Verification items for this drawing (mm, ordinates from the low corner). A direction names the side the tool comes from. Coordinates: 2 decimals unless noted, no trailing zeros. Loops run counter-clockwise (first coordinate to the right, second up) from the corner with the lowest first, then second, coordinate; pieces in that order, holes last. Notation, with made-up numbers: (47.25, 58.5) - (63.25, 58.5) arc R11 ccw to (63.25, 75.5) - close; hole circle Ø1 at (46, 4). An arc over 180 degrees is marked (long way). One line per item, written item: value. Start each with the question number.
(1) Section check D-D (y = 6). Record the boundary of the cut face in (x, z) (1 decimal), plus the area to 3 significant figures.
(2) Section check A-A (x = 150). Record the boundary of the cut face in (y, z) (1 decimal).
(3) Gauge pin test, flat ends, axial feed: P1, Ø12, axis at x = 36.5, z = 169, coming from the +Y side; P2, Ø4, axis at y = 16.5, z = 157, coming from the +X side (1 decimal); P3, Ø3, axis at y = 17.5, z = 55.5, coming from the +X side. Record the tip position at first contact, or that the pin passes through.
(4) Section check C-C (y = 26.5). Record the boundary of the cut face in (x, z) (1 decimal).
(5) Set-up check for the marked faces 4, 5 and 6: record each of +Z, -Z, +X, -X, +Y, -Y from which the full face is reachable in a straight line by a thin tool's end or side.
(6) Draft check along Z on the marked faces 1, 2 and 3. Enter one of: +Z half, -Z half, draft (parallel to the pull), parting line (faces both ways), or undercut.
(7) Thickness scan on probe 1 along Y at (x, z) = (238.5, 266.5); probe 2 along X at (y, z) = (39, 227.5); probe 3 along X at (y, z) = (5, 135.5) (1 decimal). Record the ranges inside material, lowest first. Write a range as [from, to].
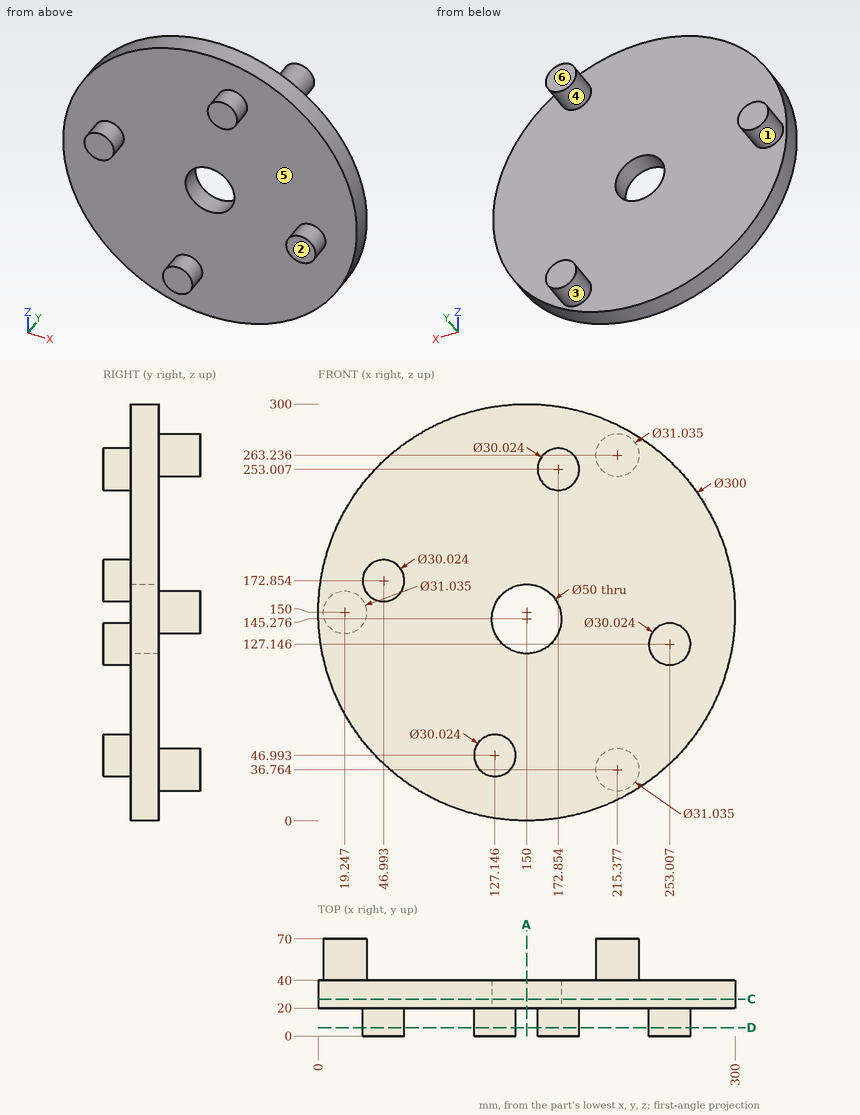
Responses:
1. outline: circle Ø30 at (47, 172.9); circle Ø30 at (127.1, 47); circle Ø30 at (172.9, 253); circle Ø30 at (253, 127.1)
1. area: 2,830 mm²
2. outline: (20, 0) - (40, 0) - (40, 120.3) - (20, 120.3) - close; (20, 170.3) - (40, 170.3) - (40, 300) - (20, 300) - close
3. P1: stops at y = 40
3. P2: stops at x = 52.8
3. P3: stops at x = 140.42
4. outline: circle Ø300 at (150, 150); hole circle Ø50 at (150, 145.3)
5. face 4: +Y
5. face 5: -Y
5. face 6: +Z, -Z, +X, -X, +Y
6. face 1: parting line
6. face 2: draft
6. face 3: undercut
7. probe 1: y = [20, 40]
7. probe 2: x = [21.57, 278.43]
7. probe 3: x = [240.5, 265.5]
